```python
from build123d import *

# Parameters (mm, degrees)
SKETCH1_W           = 140
SKETCH1_H           = 53
BOSS_EXTRUDE1_DEPTH = 38.1
BOSS_EXTRUDE2_DEPTH = 45.4
CUT_EXTRUDE1_DEPTH  = 5
BOSS_EXTRUDE3_DEPTH = 45.4
BOSS_EXTRUDE4_DEPTH = 38.1
SKETCH11_W          = 134
SKETCH11_H          = 53
CUT_EXTRUDE2_DEPTH  = 34
SKETCH12_W          = 6
SKETCH12_H          = 14
CUT_EXTRUDE3_DEPTH  = 34
SKETCH13_W          = 6
SKETCH13_H          = 5
CUT_EXTRUDE4_DEPTH  = 6
CUT_EXTRUDE6_DEPTH  = 3
CUT_EXTRUDE7_DEPTH  = 3
SKETCH17_W          = 18
SKETCH17_H          = 7
BOSS_EXTRUDE5_DEPTH = 9
SKETCH21_W          = 2
SKETCH21_H          = 12
CUT_EXTRUDE10_DEPTH = 93.075528643
SKETCH23_RX         = 3.5
SKETCH23_RY         = 1.800693379
CUT_EXTRUDE12_DEPTH = 141.213025648
FILLET3_START       = -60
FILLET3_DEPTH       = 120


with BuildPart() as part:
    # Sketch1 → Boss-Extrude1 (new body)
    with BuildSketch(Plane(origin=(0, 0, 0), x_dir=(0, 0, -1), z_dir=(1, 0, 0))):
        Rectangle(SKETCH1_W, SKETCH1_H)
    extrude(amount=BOSS_EXTRUDE1_DEPTH)

    # Sketch2 → Boss-Extrude2 (add)
    with BuildSketch(Plane(origin=(38.1, 0, 0), x_dir=(0, 0, -1), z_dir=(1, 0, 0))):
        Polygon((0, -26.5), (5, -26.5), (5, -39.566040215), (-4.99956385, -39.566040215), (-4.99956385, -26.566040215), align=None)
    extrude(amount=-BOSS_EXTRUDE2_DEPTH)

    # Sketch3 → Cut-Extrude1 (cut)
    with BuildSketch(Plane.XZ.offset(39.566040215)):
        Polygon((-5.130369, 0), (-5.130369, 2.5), (-1.130369, 2.5), (-1.130369, -2.5), (-5.130369, -2.5), align=None)
    extrude(amount=-CUT_EXTRUDE1_DEPTH, mode=Mode.SUBTRACT)

    # Sketch7 → Boss-Extrude3 (add)
    with BuildSketch(Plane(origin=(38.1, 0, 0), x_dir=(0, 0, -1), z_dir=(1, 0, 0))):
        Polygon((-4.99956385, -26.566040215), (-4.99956385, -26.5), (0, -26.5), align=None)
    extrude(amount=-BOSS_EXTRUDE3_DEPTH)

    # Sketch8 → Boss-Extrude4 (add)
    with BuildSketch(Plane(origin=(38.1, 0, 0), x_dir=(0, 0, -1), z_dir=(1, 0, 0))):
        Polygon((-70, 26.5), (-70, 32.5), (70.030085777, 32.5), (70, 26.5), align=None)
    extrude(amount=-BOSS_EXTRUDE4_DEPTH)

    # Sketch11 → Cut-Extrude2 (cut)
    with BuildSketch(Plane(origin=(38.1, 0, 0), x_dir=(0, 0, -1), z_dir=(1, 0, 0))):
        with Locations((0.007630482, 3)):
            Rectangle(SKETCH11_W, SKETCH11_H)
    extrude(amount=-CUT_EXTRUDE2_DEPTH, mode=Mode.SUBTRACT)

    # Sketch12 → Cut-Extrude3 (cut)
    with BuildSketch(Plane(origin=(38.1, 0, 0), x_dir=(0, 0, -1), z_dir=(1, 0, 0))):
        with Locations((0.000218075, -30.5)):
            Rectangle(SKETCH12_W, SKETCH12_H)
    extrude(amount=-CUT_EXTRUDE3_DEPTH, mode=Mode.SUBTRACT)

    # Sketch13 → Cut-Extrude4 (cut)
    with BuildSketch(Plane(origin=(4.1, 0, 0), x_dir=(0, 0, -1), z_dir=(1, 0, 0))):
        with Locations((0.000218075, -35)):
            Rectangle(SKETCH13_W, SKETCH13_H)
    extrude(amount=-CUT_EXTRUDE4_DEPTH, mode=Mode.SUBTRACT)

    # Sketch15 → Cut-Extrude6 (cut)
    with BuildSketch(Plane(origin=(38.1, 0, 0), x_dir=(0, 0, -1), z_dir=(1, 0, 0))):
        with BuildLine():
            ThreePointArc((-67.496184759, 31), (-68.114088128, 31.924122375), (-69.204189088, 31.706208093))
            Line((-69.204189088, 31.706208093), (-67.78818043, 30.293791907))
            ThreePointArc((-67.78818043, 30.293791907), (-67.572062384, 30.617903369), (-67.496184759, 31))
        make_face()
        with BuildLine():
            Line((-67.78818043, 30.293791907), (-69.204189088, 31.706208093))
            ThreePointArc((-69.204189088, 31.706208093), (-69.202392852, 30.291995671), (-67.78818043, 30.293791907))
        make_face()
    extrude(amount=-CUT_EXTRUDE6_DEPTH, mode=Mode.SUBTRACT)

    # Sketch16 → Cut-Extrude7 (cut)
    with BuildSketch(Plane(origin=(38.1, 0, 0), x_dir=(0, 0, -1), z_dir=(1, 0, 0))):
        with BuildLine():
            ThreePointArc((69.228596491, 31.70446537), (67.814392759, 31.709738362), (67.809119767, 30.29553463))
            Line((67.809119767, 30.29553463), (69.228596491, 31.70446537))
        make_face()
        with BuildLine():
            Line((69.228596491, 31.70446537), (67.809119767, 30.29553463))
            ThreePointArc((67.809119767, 30.29553463), (68.899818519, 30.075408641), (69.518858129, 31))
            ThreePointArc((69.518858129, 31), (69.443449488, 31.38096039), (69.228596491, 31.70446537))
        make_face()
        with BuildLine():
            ThreePointArc((69.503815241, -25), (68.887086814, -24.076364303), (67.797609438, -24.291993387))
            Line((67.797609438, -24.291993387), (69.210021043, -25.708006613))
            ThreePointArc((69.210021043, -25.708006613), (69.427450938, -25.383271573), (69.503815241, -25))
        make_face()
        with BuildLine():
            Line((69.210021043, -25.708006613), (67.797609438, -24.291993387))
            ThreePointArc((67.797609438, -24.291993387), (67.795808628, -25.706205803), (69.210021043, -25.708006613))
        make_face()
        with BuildLine():
            ThreePointArc((-67.496184759, -25), (-67.572062384, -24.617903369), (-67.78818043, -24.293791907))
            Line((-67.78818043, -24.293791907), (-69.204189088, -25.706208093))
            ThreePointArc((-69.204189088, -25.706208093), (-68.114088128, -25.924122375), (-67.496184759, -25))
        make_face()
        with BuildLine():
            Line((-69.204189088, -25.706208093), (-67.78818043, -24.293791907))
            ThreePointArc((-67.78818043, -24.293791907), (-69.202392852, -24.291995671), (-69.204189088, -25.706208093))
        make_face()
    extrude(amount=-CUT_EXTRUDE7_DEPTH, mode=Mode.SUBTRACT)

    # Sketch17 → Boss-Extrude5 (add)
    with BuildSketch(Plane.ZY):
        with Locations((49.976158348, 3)):
            Rectangle(SKETCH17_W, SKETCH17_H)
        with Locations((-49.976158348, 3)):
            Rectangle(SKETCH17_W, SKETCH17_H)
    extrude(amount=BOSS_EXTRUDE5_DEPTH)

    # Sketch21 → Cut-Extrude10 (cut, through all)
    with BuildSketch(Plane(origin=(0, 6.5, 0), x_dir=(1, 0, 0), z_dir=(0, 1, 0))):
        with Locations((-4, -49.976158348)):
            Rectangle(SKETCH21_W, SKETCH21_H)
        with Locations((-4, 49.976158348)):
            Rectangle(SKETCH21_W, SKETCH21_H)
    extrude(amount=-CUT_EXTRUDE10_DEPTH, mode=Mode.SUBTRACT)

    # Sketch23 → Cut-Extrude12 (cut, through all)
    with BuildSketch(Plane.XY.offset(58.976158348)):
        with Locations(Location((-9, 3), (0, 0, 90))):
            Ellipse(SKETCH23_RX, SKETCH23_RY)
    extrude(amount=-CUT_EXTRUDE12_DEPTH, mode=Mode.SUBTRACT)

    # Fillet3: read off the stored shape, not the designer's step
    # Fillet3 outline → Fillet3 (cut)
    with BuildSketch(Plane.XY.offset(FILLET3_START)):
        with BuildLine():
            ThreePointArc((-7.452330452, -0.5), (-7.891056374, -0.239832369), (-7.873213162, 0.269921739))
            add(Edge.make_bspline(
                [(-9, -0.5), (-8.366981638, -0.5), (-7.873213162, 0.269921739)],
                knots=[3.141592654, 3.141592654, 3.141592654, 3.823261415, 3.823261415, 3.823261415], degree=2, weights=[1, 0.872894942, 0.856107875]))
            Line((-9, -0.5), (-7.452330452, -0.5))
        make_face()
        with BuildLine():
            add(Edge.make_bspline(
                [(-7.873213161, 5.730078261), (-8.366981638, 6.5), (-9, 6.5)],
                knots=[5.601516546, 5.601516546, 5.601516546, 6.283185307, 6.283185307, 6.283185307], degree=2, weights=[0.856107875, 0.872894942, 1]))
            ThreePointArc((-7.873213161, 5.730078261), (-7.891056374, 6.239832369), (-7.452330452, 6.5))
            Line((-7.452330452, 6.5), (-9, 6.5))
        make_face()
    extrude(amount=FILLET3_DEPTH, mode=Mode.SUBTRACT)


solid = part.part
```
Source: CAD feature listing. Evaluate the final solid. Frame: model axes, mm. A direction names the side the tool comes from. Round coordinates to 2 decimals unless told otherwise and drop trailing zeros. Loops run counter-clockwise (first coordinate to the right, second up) from the corner with the lowest first, then second, coordinate; pieces in that order, holes last.
(1) Section query B-B (y = -3.5). Output: boundary loops of the cut face in (x, z), and give its area (3 significant figures).
From the geometry:
outline: (0, -70) - (38.1, -70) - (38.1, -67.01) - (4.1, -67.01) - (4.1, 66.99) - (38.1, 66.99) - (38.1, 70) - (0, 70) - close
area: 778 mm2
(2) Section query C-C (z = 32.5). Output: boundary loops of the cut face in (x, y), and give its area (3 significant figures).
From the geometry:
outline: (0, -26.5) - (38.1, -26.5) - (38.1, -23.5) - (4.1, -23.5) - (4.1, 29.5) - (38.1, 29.5) - (38.1, 32.5) - (0, 32.5) - close
area: 446 mm2
(3) Contact query for flat-ended pins moving along their axis: pin 1 Ø3.5 at (x, z) = (-4, 50) entering from -Y; pin 2 Ø6.5 at (x, y) = (15, -34.5) entering from +Z; pin 3 Ø1.5 at (x, z) = (5.5, -22) entering from -Y. Output: stop coordinate, or through.
From the geometry:
pin 1: stops at y = -0.5
pin 2: stops at z = 5
pin 3: stops at y = -26.5
(4) Material intervals for probe 1 along Y at (x, z) = (31.5, 43); probe 2 along Z at (x, y) = (26.5, 15); probe 3 along Y at (x, z) = (36.5, 4.5), sorted ascending.
From the geometry:
probe 1: y = -26.5 to -23.5, 29.5 to 32.5
probe 2: z = -70 to -67.01, 66.99 to 70
probe 3: y = -39.57 to -23.5, 29.5 to 32.5
(5) Pull-direction query (Y, two-part tool) for faces 5 (the flat face through (21, -23.5, 35)), 6 (the flat face through (19, -26.5, -37)), 7 (the flat face through (-2.8, 6.5, 49.9)), 8 (the flat face through (-3, -37, -2.5)); classes: +Y half, -Y half, draft (parallel to the pull), parting line (faces both ways), or undercut.
From the geometry:
face 5: undercut
face 6: -Y half
face 7: +Y half
face 8: draft
(6) Section query A-A (x = 33). Output: boundary loops of the cut face in (y, z).
From the geometry:
outline: (-39.57, -5) - (-26.5, -5) - (-26.5, -70) - (26.5, -70) - (32.5, -70.03) - (32.5, 70) - (-26.5, 70) - (-26.5, 5) - (-39.57, 5) - close; hole (-37.5, -3) - (-23.5, -3) - (-23.5, -67.01) - (29.5, -67.01) - (29.5, 66.99) - (-23.5, 66.99) - (-23.5, 3) - (-37.5, 3) - close
(7) Access query for faces 1 (the flat face through (-3, 3, -50)), 2 (the flat face through (-5.13, -37, 0)), 3 (the flat face through (-2.8, -0.5, 49.9)), 4 (the flat face through (18, -31, 3)). Directions: +Z, -Z, +X, -X, +Y, -Y. A direction counts if a zero-diameter tool reaches every point of the face in a straight line with its end or side. Return the directions, or none.
From the geometry:
face 1: +Y, -Y
face 2: -Y
face 3: +Z, -Z, -X, -Y
face 4: +X
